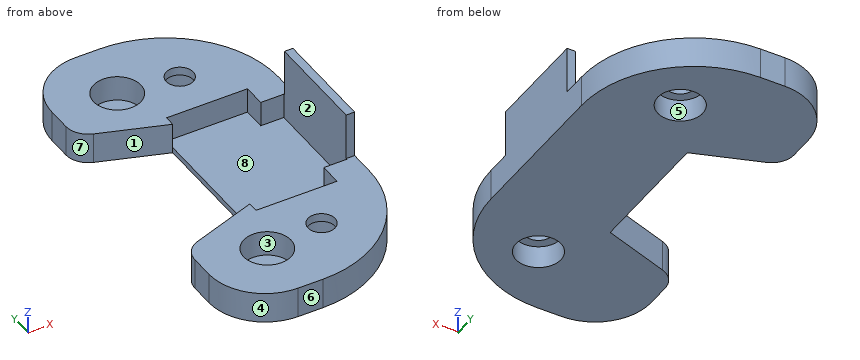
from build123d import *

# Parameters (mm, degrees)
F0_R      = 2.1
F1_DEPTH  = 2.75
F2_W      = 13.5
F2_H      = 2.25
F3_DEPTH  = 10
F4_W      = 2.8
F4_H      = 2
F5_DEPTH  = 2.25
F6_R      = 10
F7_R      = 2
F8_R      = 2
F9_DEPTH  = 2
F10_R     = 1.2
F11_R     = 1.2
F12_DEPTH = 0.75
F13_W     = 0.75
F13_H     = 9.5
F14_DEPTH = 2.25
F15_W     = 0.75
F15_H     = 9.5
F16_DEPTH = 4.2
F17_R     = 2.1
F18_DEPTH = 0.5
F19_W     = 0.75
F19_H     = 0.1
F20_DEPTH = 4.2


with BuildPart() as f1:
    # F0 (on Top) → F1 (new body)
    with BuildSketch(Plane.XY):
        with BuildLine():
            Line((11.6860830059, 16.8135), (5.5, 16.8135))
            Line((5.5, 16.8135), (-0.5, 16.8135))
            ThreePointArc((-0.5, 16.8135), (-4.0355339059, 15.3490339059), (-5.5, 11.8135))
            Line((-5.5, 11.8135), (-5.5, 8.3135))
            Line((-5.5, 8.3135), (1.6860830059, 5.8135))
            Line((1.6860830059, 5.8135), (1.6860830059, -5.814))
            Line((1.6860830059, -5.814), (-5.5, -8.314))
            Line((-5.5, -8.314), (-5.5, -11.814))
            ThreePointArc((-5.5, -11.814), (-4.0355339059, -15.3495339059), (-0.5, -16.814))
            Line((-0.5, -16.814), (5.5, -16.814))
            Line((5.5, -16.814), (11.6860830059, -16.814))
            Line((11.6860830059, -16.814), (11.6860830059, 16.8135))
        make_face()
        with Locations((0, -11.314)):
            Circle(F0_R, mode=Mode.SUBTRACT)
        with Locations((0, 11.3135)):
            Circle(F0_R, mode=Mode.SUBTRACT)
    extrude(amount=F1_DEPTH)

    # F2 (on face) → F3 (cut, through all)
    with BuildSketch(Plane.YZ.offset(11.6860830059)):
        with Locations((0, 1.625)):
            Rectangle(F2_W, F2_H)
    extrude(amount=-F3_DEPTH, mode=Mode.SUBTRACT)

    # F4 (on face) → F5 (join, through all)
    with BuildSketch(Plane.XY.offset(0.5)):
        with Locations((10.2860830059, -5.75)):
            Rectangle(F4_W, F4_H)
        with Locations((10.2860830059, 5.75)):
            Rectangle(F4_W, F4_H)
    extrude(amount=F5_DEPTH)

    # F6
    f6_edges = [f1.edges().sort_by_distance(p)[0] for p in [
        (11.686083, -16.814, 1.375),
        (11.686083, 16.8135, 1.375),
    ]]
    fillet(f6_edges, radius=F6_R)

    # F7
    f7_edges = [f1.edges().sort_by_distance(p)[0] for p in [
        (-5.5, -8.314, 1.375),
        (-5.5, 8.3135, 1.375),
    ]]
    fillet(f7_edges, radius=F7_R)

    # F8 (on face) → F9 (cut)
    with BuildSketch(Plane(origin=(0, 0, 0), x_dir=(1, 0, 0), z_dir=(0, 0, -1))):
        with Locations((5.1860830059, -10.6868971724)):
            Circle(F8_R)
        with Locations((5.1860830059, 10.6873971724)):
            Circle(F8_R)
    extrude(amount=-F9_DEPTH, mode=Mode.SUBTRACT)

    # F10 (on face) + F11 (on face) → F12 (cut, through all)
    with BuildSketch(Plane(origin=(0, 0, 2), x_dir=(1, 0, 0), z_dir=(0, 0, -1))):
        with Locations((5.1860830059, -10.6868971724)):
            Circle(F10_R)
    with BuildSketch(Plane(origin=(0, 0, 2), x_dir=(1, 0, 0), z_dir=(0, 0, -1))):
        with Locations((5.1860830059, 10.6873971724)):
            Circle(F11_R)
    extrude(amount=-F12_DEPTH, mode=Mode.SUBTRACT)

    # F13 (on face) → F14 (join, through all)
    with BuildSketch(Plane.XY.offset(0.5)):
        with Locations((11.3110830059, 0)):
            Rectangle(F13_W, F13_H)
    extrude(amount=F14_DEPTH)

    # F15 (on face) → F16 (join)
    with BuildSketch(Plane.XY.offset(2.75)):
        with Locations((11.3110830059, 0)):
            Rectangle(F15_W, F15_H)
    extrude(amount=F16_DEPTH)

    # F17 (on face) → F18 (join)
    with BuildSketch(Plane(origin=(0, 0, 0), x_dir=(1, 0, 0), z_dir=(0, 0, -1))):
        with Locations((0, 11.314)):
            Circle(F17_R)
        with Locations((0, -11.3135)):
            Circle(F17_R)
    extrude(amount=-F18_DEPTH)

    # F19 (on face) → F20 (cut, through all)
    with BuildSketch(Plane.XY.offset(6.95)):
        with Locations((11.3110830059, 4.7)):
            Rectangle(F19_W, F19_H)
        with Locations((11.3110830059, -4.7)):
            Rectangle(F19_W, F19_H)
    extrude(amount=-F20_DEPTH, mode=Mode.SUBTRACT)


solid = f1.part
For this review, take the finished solid that the model builds, in its own axes (mm). Face numbers are marked on the shaded views. A direction names the side the tool comes from. Round coordinates to 2 decimals unless told otherwise and drop trailing zeros. Loops run counter-clockwise (first coordinate to the right, second up) from the corner with the lowest first, then second, coordinate; pieces in that order, holes last. Notation, with made-up numbers: (-0.5, -25) - (44.5, -25) arc R26 cw to (44.5, -2) - close; hole circle Ø2 at (-1, -18.5). An arc over 180 degrees is marked (long way). One line per item, written item: value. Start each with the question number.
Item 1: Take a section at D-D (x = 2.5). Give the boundary of the cut face in (y, z), plus the area to 3 significant figures.
Item 2: For L1, parallel to Y at x = 0, z = 1.1; L2, parallel to Z at x = 2.5, y = -12; L3, parallel to Z at x = 8.25, y = 6.5, list the stretches that pass through material, from the lowest coordinate up.
Item 3: Take a section at C-C (z = 1). Give the boundary of the cut face in (x, y).
Item 4: Take a section at B-B (y = 0). Give the boundary of the cut face in (x, z), plus the area to 3 significant figures.
Item 5: Take a section at A-A (x = 0). Give the boundary of the cut face in (y, z), plus the area to 3 significant figures.
Item 6: For the marked faces 1, 2, 3, 4 and 5, list the 3-axis set-ups (+Z, -Z, +X, -X, +Y, -Y) from which the entire face can be reached by the end or side of a thin tool; tool diameter is ignored.
Item 7: The part is to be moulded in two halves that separate along X. For the marked faces 6, 7 and 8, say which applies: +X half, -X half, draft (parallel to the pull), parting line (faces both ways), or undercut.
Item 8: Clearance check with flat-ended pins moving along their axes: pin 1 Ø5 at (x, y) = (-2, -6.5) entering from +Z; pin 2 Ø1.9 at (x, y) = (5.19, 10.69) entering from +Z; pin 3 Ø2.5 at (x, z) = (10, 2) entering from +Y; pin 4 Ø0.7 at (x, z) = (5.5, 1) entering from -Y. State where each tip first meets the part, or that it passes through.
Answer below:
1. outline: (-16.78, 0) - (16.78, 0) - (16.78, 2.75) - (6.75, 2.75) - (6.75, 0.5) - (-6.75, 0.5) - (-6.75, 2.75) - (-16.78, 2.75) - close
1. area: 61.9 mm2
2. L1: y = -16.81 to -13.41, -9.21 to -6.4, 6.4 to 9.21, 13.41 to 16.81
2. L2: z = 0 to 2.75
2. L3: z = 0 to 0.5
3. outline: (-5.5, -11.81) arc R5 ccw to (-0.5, -16.81) - (1.69, -16.81) arc R10 ccw to (11.69, -6.81) - (11.69, 6.81) arc R10 ccw to (1.69, 16.81) - (-0.5, 16.81) arc R5 ccw to (-5.5, 11.81) - (-5.5, 9.74) arc R2 ccw to (-4.16, 7.85) - (1.69, 5.81) - (1.69, 6.75) - (8.89, 6.75) - (8.89, 4.75) - (10.94, 4.75) - (10.94, -4.75) - (8.89, -4.75) - (8.89, -6.75) - (1.69, -6.75) - (1.69, -5.81) - (-4.16, -7.85) arc R2 ccw to (-5.5, -9.74) - close; hole circle Ø4.2 at (0, -11.31); hole circle Ø4.2 at (0, 11.31); hole circle Ø4 at (5.19, -10.69); hole circle Ø4 at (5.19, 10.69)
4. outline: (1.69, 0) - (11.69, 0) - (11.69, 6.95) - (10.94, 6.95) - (10.94, 0.5) - (1.69, 0.5) - close
4. area: 9.84 mm2
5. outline: (-16.81, 0) - (-6.4, 0) - (-6.4, 2.75) - (-9.21, 2.75) - (-9.21, 0.5) - (-13.41, 0.5) - (-13.41, 2.75) - (-16.81, 2.75) - close; (6.4, 0) - (16.81, 0) - (16.81, 2.75) - (13.41, 2.75) - (13.41, 0.5) - (9.21, 0.5) - (9.21, 2.75) - (6.4, 2.75) - close
5. area: 38.4 mm2
6. face 1: +Z, -Z, -X
6. face 2: +Z, -X
6. face 3: +Z
6. face 4: +Z, -Z, -X, -Y
6. face 5: -Z
7. face 6: draft
7. face 7: -X half
7. face 8: undercut
8. pin 1: stops at z = 2.75
8. pin 2: passes through
8. pin 3: stops at y = 13.89
8. pin 4: stops at y = -16.19
